Verification items for the finished model (mm, model axes). Face numbers are marked on the shaded views. A direction names the side the tool comes from. Coordinates: 2 decimals unless noted, no trailing zeros. Loops run counter-clockwise (first coordinate to the right, second up) from the corner with the lowest first, then second, coordinate; pieces in that order, holes last. Notation, with made-up numbers: (48.5, 46.5) -> (69.5, 46.5) arc R24 ccw to (69.5, 71.5) -> close; hole circle Ø4 at (25, 66.25). An arc over 180 degrees is marked (long way). Answer as a JSON object with one key per item and string values. Group by question number.
Q1. Release check for a two-part mould opening along X. For the marked faces 1, 2 and 3 record: released by +X, released by -X, zero draft, split by the parting line, or undercut.
Q2. Cross-section at B-B on y = 49.5. Record the boundary of the cut face in (x, z).
Q3. Scan lines: L1, parallel to X at y = 24, z = 9; L2, parallel to X at y = 31, z = 21; L3, parallel to Y at x = -39, z = 28. Record each from-to range of solid material in increasing order.
Q4. Set-up check for the marked faces 4, 5 and 6: record each of +Z, -Z, +X, -X, +Y, -Y from which the full face is reachable in a straight line by a thin tool's end or side.
Q5. Gauge pin test, flat ends, axial feed: pin 1 Ø10 at (x, y) = (2, 29) entering from +Z; pin 2 Ø3 at (x, z) = (-1.5, 0.5) entering from -Y; pin 3 Ø1 at (x, z) = (-37, 10) entering from -Y; pin 4 Ø1.6 at (x, y) = (-29.27, 18.51) entering from +Z. Record the tip position at first contact, or that the pin passes through.
Q6. Cross-section at D-D on z = 5. Record the boundary of the cut face in (x, y).
Q7. Cross-section at A-A on z = 23. Record the boundary of the cut face in (x, y), and give its area (3 significant figures).
Q8. Cross-section at C-C on z = 12.25. Record the boundary of the cut face in (x, y), and give its area (3 significant figures).
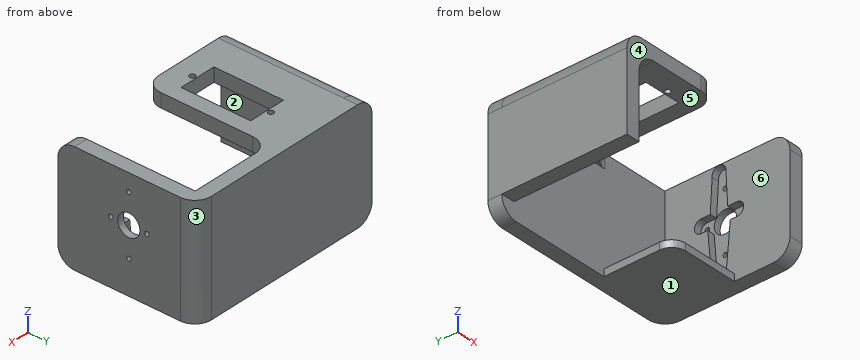
```python
from build123d import *

# Parameters (mm, degrees)
EXTRUDE_1_DEPTH     = 40
FILLET_2_R          = 6
FILLET_3_R          = 6
FILLET_4_R          = 6
FILLET_5_R          = 6
FILLET_6_R          = 6
CUT_EXTRUDE_1_DEPTH = 2.6
EXTRUDE_START       = 45
EXTRUDE_2_DEPTH     = 45
SKETCH_4_R          = 1
SKETCH_4_W          = 13.5
SKETCH_4_H          = 25
CUT_EXTRUDE_2_DEPTH = 60
FILLET_7_R          = 6
FILLET_8_R          = 6
SKETCH_5_R          = 0.8
SKETCH_5_R_2        = 4
CUT_EXTRUDE_3_DEPTH = 10
EXTRUDE_START_2     = -2.5
EXTRUDE_4_DEPTH     = 2.5
FILLET_9_R          = 5


with BuildPart() as part:
    # 草图1 → 凸台-拉伸1 (new body)
    with BuildSketch(Plane.XY):
        Polygon((12.980970113, 56.471676883), (12.980970113, 11.471676883), (17.980970113, 11.471676883), (17.980970113, 61.471676883), (-54.019029887, 61.471676883), (-54.019029887, 56.471676883), (-49.554341186, 56.471676883), align=None)
    extrude(amount=EXTRUDE_1_DEPTH)

    # 圆角2
    fillet_2_edges = [part.edges().sort_by_distance(p)[0] for p in [
        (17.980970113, 61.471676883, 20),
    ]]
    fillet(fillet_2_edges, radius=FILLET_2_R)

    # 圆角3
    fillet_3_edges = [part.edges().sort_by_distance(p)[0] for p in [
        (15.480970113, 11.471676883, 0),
    ]]
    fillet(fillet_3_edges, radius=FILLET_3_R)

    # 圆角4
    fillet_4_edges = [part.edges().sort_by_distance(p)[0] for p in [
        (15.480970113, 11.471676883, 40),
    ]]
    fillet(fillet_4_edges, radius=FILLET_4_R)

    # 圆角5
    fillet_5_edges = [part.edges().sort_by_distance(p)[0] for p in [
        (-54.019029887, 58.971676883, 0),
    ]]
    fillet(fillet_5_edges, radius=FILLET_5_R)

    # 圆角6
    fillet_6_edges = [part.edges().sort_by_distance(p)[0] for p in [
        (-54.019029887, 58.971676883, 40),
    ]]
    fillet(fillet_6_edges, radius=FILLET_6_R)

    # 草图2 → 切除-拉伸1 (cut)
    with BuildSketch(Plane.ZY.offset(-12.980970113)):
        with BuildLine():
            Line((25.4, 43.428225459), (25.4, 40.117895335))
            Line((25.4, 40.117895335), (37.115774764, 39.455783428))
            ThreePointArc((37.115774764, 39.455783428), (39.95, 36.978225459), (37.115774764, 34.500667489))
            Line((37.115774764, 34.500667489), (25.4, 33.838555582))
            Line((25.4, 33.838555582), (25.4, 30.528225459))
            ThreePointArc((25.4, 30.528225459), (23, 28.128225459), (20.6, 30.528225459))
            Line((20.6, 30.528225459), (20.6, 32.921208444))
            Line((20.6, 32.921208444), (5.903894821, 34.243983881))
            ThreePointArc((5.903894821, 34.243983881), (3.404704977, 36.978225459), (5.903894821, 39.712467036))
            Line((5.903894821, 39.712467036), (20.6, 41.035242473))
            Line((20.6, 41.035242473), (20.6, 43.428225459))
            ThreePointArc((20.6, 43.428225459), (23, 45.828225459), (25.4, 43.428225459))
        make_face()
    extrude(amount=-CUT_EXTRUDE_1_DEPTH, mode=Mode.SUBTRACT)

    # 草图3 → 凸台-拉伸2 (add)
    with BuildSketch(Plane.XZ.offset(-56.471676883).offset(EXTRUDE_START)):
        with BuildLine():
            Line((-54.019029887, 34), (-54.019029887, 6))
            Line((-54.019029887, 6), (-49.019029887, 6))
            Line((-49.019029887, 6), (-49.019029887, 29))
            ThreePointArc((-49.019029887, 29), (-47.261670574, 33.242640687), (-43.019029887, 35))
            Line((-43.019029887, 35), (-17.519029887, 35))
            Line((-17.519029887, 35), (-17.519029887, 40))
            Line((-17.519029887, 40), (-48.019029887, 40))
            ThreePointArc((-48.019029887, 40), (-52.261670574, 38.242640687), (-54.019029887, 34))
        make_face()
    extrude(amount=-EXTRUDE_2_DEPTH)

    # 草图4 → 切除-拉伸2 (cut)
    with BuildSketch(Plane.XY.offset(40)):
        with Locations((-29.269029887, 18.508506795)):
            Circle(SKETCH_4_R)
        with Locations((-29.769029887, 46.304010029)):
            Circle(SKETCH_4_R)
        with Locations((-29.769029887, 32.408506795)):
            Rectangle(SKETCH_4_W, SKETCH_4_H)
    extrude(amount=-CUT_EXTRUDE_2_DEPTH, mode=Mode.SUBTRACT)

    # 圆角7
    fillet_7_edges = [part.edges().sort_by_distance(p)[0] for p in [
        (-17.519029887, 11.471676883, 37.5),
    ]]
    fillet(fillet_7_edges, radius=FILLET_7_R)

    # 圆角8
    fillet_8_edges = [part.edges().sort_by_distance(p)[0] for p in [
        (-17.519029887, 56.471676883, 37.5),
    ]]
    fillet(fillet_8_edges, radius=FILLET_8_R)

    # 草图5 → 切除-拉伸3 (cut)
    with BuildSketch(Plane.ZY.offset(-15.580970113)):
        with Locations(Location((12.25, 36.978225459, 0), (0, 0, 270))):
            Circle(SKETCH_5_R)
        with Locations(Location((23, 36.978225459, 0), (0, 0, 270))):
            Circle(SKETCH_5_R_2)
        with Locations(Location((33.75, 36.978225459, 0), (0, 0, 270))):
            Circle(SKETCH_5_R)
        with Locations(Location((23, 30.478225459, 0), (0, 0, 270))):
            Circle(SKETCH_5_R)
        with Locations(Location((23, 43.478225459, 0), (0, 0, 270))):
            Circle(SKETCH_5_R)
    extrude(amount=-CUT_EXTRUDE_3_DEPTH, mode=Mode.SUBTRACT)

    # 草图7 → 凸台-拉伸4 (add)
    with BuildSketch(Plane(origin=(0, 0, 0), x_dir=(-1, 0, 0), z_dir=(0, 0, -1)).offset(EXTRUDE_START_2)):
        with BuildLine():
            Line((-17.980970113, 55.471676883), (-17.980970113, 31.471676883))
            Line((-17.980970113, 31.471676883), (12.019029887, 31.471676883))
            Line((12.019029887, 31.471676883), (12.019029887, 61.471676883))
            Line((12.019029887, 61.471676883), (-11.980970113, 61.471676883))
            ThreePointArc((-11.980970113, 61.471676883), (-16.2236108, 59.71431757), (-17.980970113, 55.471676883))
        make_face()
    extrude(amount=EXTRUDE_4_DEPTH)

    # 圆角9
    fillet_9_edges = [part.edges().sort_by_distance(p)[0] for p in [
        (-12.019029887, 31.471676883, 1.25),
    ]]
    fillet(fillet_9_edges, radius=FILLET_9_R)


solid = part.part
```
Computed values:
{
 "1": {"face 1": "zero draft", "face 2": "undercut", "face 3": "released by +X"},
 "2": {"outline": "(-54.02, 6) -> (-49.02, 6) -> (-49.02, 29) arc R6 cw to (-43.02, 35) -> (-17.52, 35) -> (-17.52, 40) -> (-48.02, 40) arc R6 ccw to (-54.02, 34) -> close; (-12.02, 0) -> (17.98, 0) -> (17.98, 40) -> (12.98, 40) -> (12.98, 2.5) -> (-12.02, 2.5) -> close"},
 "3": {"L1": "x = -54.02 to -49.02, 12.98 to 17.98", "L2": "x = -54.02 to -49.02, 15.58 to 17.98", "L3": "y = 56.47 to 61.47"},
 "4": {"face 4": "+Z, -Z, +X, -X, -Y", "face 5": "-Z, -Y", "face 6": "+Z, -Y"},
 "5": {"pin 1": "stops at z = 2.5", "pin 2": "stops at y = 31.47", "pin 3": "stops at y = 56.47", "pin 4": "passes through"},
 "6": {"outline": "(-53.94, 56.47) -> (12.98, 56.47) -> (12.98, 39.47) -> (15.58, 39.47) -> (15.58, 34.49) -> (12.98, 34.49) -> (12.98, 11.56) -> (17.98, 11.56) -> (17.98, 55.47) arc R6 ccw to (11.98, 61.47) -> (-53.94, 61.47) -> close"},
 "7": {"outline": "(-54.02, 11.47) -> (-49.02, 11.47) -> (-49.02, 56.47) -> (12.98, 56.47) -> (12.98, 45.83) -> (15.58, 45.83) -> (15.58, 44.28) -> (17.98, 44.28) -> (17.98, 55.47) arc R6 ccw to (11.98, 61.47) -> (-54.02, 61.47) -> close; (12.98, 11.47) -> (17.98, 11.47) -> (17.98, 29.68) -> (15.58, 29.68) -> (15.58, 28.13) -> (12.98, 28.13) -> close; (15.58, 31.28) -> (17.98, 31.28) -> (17.98, 32.98) -> (15.58, 32.98) -> close; (15.58, 40.98) -> (17.98, 40.98) -> (17.98, 42.68) -> (15.58, 42.68) -> close", "area": "729 mm²"},
 "8": {"outline": "(-54.02, 11.47) -> (-49.02, 11.47) -> (-49.02, 56.47) -> (12.98, 56.47) -> (12.98, 40.28) -> (15.58, 40.28) -> (15.58, 37.78) -> (17.98, 37.78) -> (17.98, 55.47) arc R6 ccw to (11.98, 61.47) -> (-54.02, 61.47) -> close; (12.98, 11.47) -> (17.98, 11.47) -> (17.98, 36.18) -> (15.58, 36.18) -> (15.58, 33.67) -> (12.98, 33.67) -> close", "area": "781 mm²"}
}
